For this review, take the finished solid that the model builds, in its own axes (mm). A direction names the side the tool comes from. Coordinates: 2 decimals unless noted, no trailing zeros. Loops run counter-clockwise (first coordinate to the right, second up) from the corner with the lowest first, then second, coordinate; pieces in that order, holes last.
1. Take a section at C-C, the plane x = 11.75. State the section outline as (y, z) points, then the cut area to 3 significant figures.
2. To check wall thickness, follow probe 1 along Z at (x, y) = (0, -11.35); probe 2 along Z at (x, y) = (0, -4.25); probe 3 along X at (y, z) = (6.3, 0). State the ranges of each line that lie inside material, in increasing order.
3. Take a section at A-A, the plane y = -7.5. State the section outline as (x, z) points, then the cut area to 3 significant figures.
4. Take a section at D-D, the plane z = -11.5. State the section outline as (x, y) points.
5. Mouldability with a two-part tool opening along X and no side actions: class faces 1 (the face through (1, -6, 8)), 2 (the face through (1.43, 5.52, 2.75)), 3 (the face through (-7.493, -1.479, -0.33)) as pulls with the +X half, pulls with the -X half, needs draft (parallel to the pull), parting line crosses it, or undercut.
6. Take a section at B-B, the plane z = 8.25. State the section outline as (x, y) points.
7. Machinability: for faces 4 (the face through (4.38, -6.99, 8.43)), 5 (the face through (-7.493, -4.986, -0.33)), 6 (the face through (-0.54, -10.99, 2.44)), which of the approach directions +Z, -Z, +X, -X, +Y, -Y give a long, thin tool a straight path to every point of the face, cutting with its end or side? Answer none if there is none.
8. Clearance check with flat-ended pins moving along their axes: P1, Ø8, axis at x = -8, y = 2.5, coming from the -Z side; P2, Ø2.5, axis at x = -0.5, z = -1.5, coming from the +Y side; P3, Ø5, axis at y = -1.5, z = -7.5, coming from the +X side; P4, Ø3, axis at x = 0.5, z = 0.5, coming from the +Y side. State where each tip first meets the part, or that it passes through.
Autodesk Inventor part; units mm, degrees
ref_plane "РабПлоскость1" through (-11.6426, -12, -11.6426) normal (0, -1, 0) x (1, 0, 0)
ref_plane "РабПлоскость2" through (-5.2921, -22, -5.2921) normal (0, -1, 0) x (1, 0, 0)
ref_plane "РабПлоскость3" through (-15.9179, 7, -15.9179) normal (0, 1, 0) x (0.0632, 0, 0.998)
sketch "Эскиз1" plane through (0, 0, 0) normal (0, 1, 0) x (-1, 0, 0)
  circle A0 centre (0, 0) radius 9.5
  dimension "d0" = 19
extrude "Выдавливание1" add sketch "Эскиз1" along normal blind 5
sketch "Эскиз2" plane through (0, 0, 0) normal (0, -1, 0) x (1, 0, 0)
  circle A0 centre (0, 0) radius 7.5
  dimension "d3" = 15
extrude "Выдавливание2" add sketch "Эскиз2" along normal blind 3
sketch "Эскиз3" plane through (0, -3, 0) normal (0, -1, 0) x (1, 0, 0)
  circle A0 centre (0, 0) radius 9.5
  dimension "d15" = 19
extrude "Выдавливание3" add sketch "Эскиз3" along normal blind 1
sketch "Эскиз4" plane through (0, -4, 0) normal (0, -1, 0) x (1, 0, 0)
  circle A0 centre (0, 0) radius 7.5
  dimension "d17" = 15
extrude "Выдавливание4" add sketch "Эскиз4" along normal blind 2
sketch "Эскиз5" plane through (0, -6, 0) normal (0, -1, 0) x (1, 0, 0)
  circle A0 centre (0, 0) radius 9.5
  dimension "d16" = 19
extrude "Выдавливание5" add sketch "Эскиз5" along normal blind 2
sketch "Эскиз8" plane through (0, -8, 0) normal (0, -1, 0) x (1, 0, 0)
  circle A0 centre (0, 0) radius 15
  dimension "d21" = 30
extrude "Выдавливание8" add sketch "Эскиз8" along normal blind 2
sketch "Эскиз6" plane through (0, 5, 0) normal (0, 1, 0) x (1, 0, 0)
  circle A0 centre (0, 0) radius 2.6
  dimension "d12" = 5.2
extrude "Выдавливание6" cut sketch "Эскиз6" against normal blind 27
sketch "Эскиз10" plane through (0, -10, 0) normal (0, -1, 0) x (1, 0, 0)
  circle A0 centre (0, 0) radius 15
  circle A1 centre (0, 0) radius 15
  circle A2 centre (0, 0) radius 2.5
  circle A3 centre (0, 0) radius 2.5
ref_plane "РабПлоскость1" through (-11.6426, -12, -11.6426) normal (0, -1, 0) x (1, 0, 0)
extrude "Выдавливание10" add sketch "Эскиз10" along normal up to surface (2 mm away)
sketch "Эскиз11" plane through (0, -12, 0) normal (0, -1, 0) x (1, 0, 0)
  circle A0 centre (0, 0) radius 5
  circle A1 centre (0, 0) radius 5
  circle A2 centre (0, 0) radius 2.7
  point P0 (0, 0)
  dimension "d38" = 5.4
ref_plane "РабПлоскость2" through (-5.2921, -22, -5.2921) normal (0, -1, 0) x (1, 0, 0)
sketch "Эскиз13" plane through (0, 5, 0) normal (0, 1, 0) x (1, 0, 0)
  circle A0 centre (0, 0) radius 9.5
ref_plane "РабПлоскость3" through (-15.9179, 7, -15.9179) normal (0, 1, 0) x (0.0632, 0, 0.998)
extrude "Выдавливание14" add sketch "Эскиз13" along normal up to surface (2 mm away)
sketch "Эскиз14" plane through (0, 7, 0) normal (0, 1, 0) x (1, 0, 0)
  circle A0 centre (0, 0) radius 3.1
  dimension "d48" = 6.2
extrude "Выдавливание15" cut sketch "Эскиз14" against normal blind 3
properties part number "диск"
Results list:
1. outline: (-12, -9.32) - (-8, -9.32) - (-8, 9.32) - (-12, 9.32) - close
1. area: 74.6 mm2
2. probe 1: z = -15 to -2.5, 2.5 to 15
2. probe 2: z = -7.5 to -2.6, 2.6 to 7.5
2. probe 3: x = -9.5 to -3.1, 3.1 to 9.5
3. outline: circle Ø19 at (0, 0); hole circle Ø5.2 at (0, 0)
3. area: 262 mm2
4. outline: (-9.63, -12) - (9.63, -12) - (9.63, -8) - (-9.63, -8) - close
5. face 1: needs draft
5. face 2: undercut
5. face 3: parting line crosses it
6. outline: (-12.53, -12) - (12.53, -12) - (12.53, -8) - (4.71, -8) - (4.71, -6) - (-4.71, -6) - (-4.71, -8) - (-12.53, -8) - close; (-4.71, -4) - (4.71, -4) - (4.71, -3) - (-4.71, -3) - close; (-4.71, 0) - (4.71, 0) - (4.71, 7) - (-4.71, 7) - close
7. face 4: +Y
7. face 5: none
7. face 6: +Y, -Y
8. P1: stops at z = -8.62
8. P2: stops at y = 4
8. P3: stops at x = 7.75
8. P4: passes through
